Source: CAD feature listing. Evaluate the final solid. Frame: model axes, mm. A direction names the side the tool comes from. Coordinates: 2 decimals unless noted, no trailing zeros. Write each loop counter-clockwise with the first axis right and the second up, starting at its lowest first coordinate (ties: lowest second). Pieces come first, ordered by that corner, then holes. Notation, with made-up numbers: (48, -25.75) -> (87, -25.75) arc R9 ccw to (87, -12.75) -> close; hole circle Ø1 at (-33.5, 8). An arc over 180 degrees is marked (long way). One line per item, written item: value. Start each with the question number.
1. Line query: line 1 (Y direction, x = 10, z = 11); line 2 (X direction, y = 13.6, z = 0); line 3 (Z direction, x = 9, y = 7). Output: solid intervals per line, ascending.
2. First-contact query: P1, Ø2, axis at x = -3, z = 36.5, coming from the -Y side; P2, Ø7, axis at x = 0, z = 0, coming from the +Y side; P3, Ø5.5, axis at x = 3.5, z = 39, coming from the +Y side; P4, Ø4, axis at x = -9.5, y = 6.5, coming from the -Z side. Flat tips, straight axial feed; report the tip coordinate or a pass-through.
3. Section query A-A, the plane y = -0.5. Output: boundary loops of the cut face in (x, z), and give its area (3 significant figures).
4. Section query D-D, the plane z = -3. Output: boundary loops of the cut face in (x, y), and give its area (3 significant figures).
5. Section query B-B, the plane x = 0. Output: boundary loops of the cut face in (y, z), and give its area (3 significant figures).
6. Section query C-C, the plane z = -11. Output: boundary loops of the cut face in (x, y), and give its area (3 significant figures).
7. Access query for faces 4 (the flat face through (0, 12, 5)), 5 (the cylindrical face through (0, 0, 38)), 6 (the flat face through (-0.6, 4, 39.3)). Directions: +Z, -Z, +X, -X, +Y, -Y. A direction counts if a zero-diameter tool reaches every point of the face in a straight line with its end or side. Return the directions, or none.
8. Mould query, pull axis X, two halves, no side actions, for faces 1 (the flat face through (-0.6, -4, 39.3)), 2 (the cylindrical face through (0, 14, -15)), 3 (the cylindrical face through (-3.905, -13.972, -0.867)). Classes: released by +X, released by -X, zero draft, split by the parting line, or undercut.
from build123d import *

# Parameters (mm, degrees)
BOSS_EXTRUDE1_START = 12
SKETCH1_R           = 4
BOSS_EXTRUDE1_DEPTH = 4
BOSS_EXTRUDE2_START = -12
SKETCH1_2_R         = 4
BOSS_EXTRUDE2_DEPTH = 4
SKETCH2_W           = 30
SKETCH2_H           = 32
BOSS_EXTRUDE3_DEPTH = 8
BOSS_EXTRUDE4_START = -12
BOSS_EXTRUDE4_DEPTH = 8
FILLET1_R           = 1


with BuildPart() as part:
    # Sketch1 → Boss-Extrude1 (new body)
    with BuildSketch(Plane(origin=(0, 0, 0), x_dir=(1, 0, 0), z_dir=(0, 1, 0)).offset(BOSS_EXTRUDE1_START)):
        with BuildLine():
            Line((-15, 0), (-15, -25))
            Line((-15, -25), (15, -25))
            Line((15, -25), (15, 0))
            ThreePointArc((15, 0), (0, 15), (-15, 0))
        make_face()
        with Locations(Location((0, 0, 0), (0, 0, 270))):
            Circle(SKETCH1_R, mode=Mode.SUBTRACT)
    extrude(amount=BOSS_EXTRUDE1_DEPTH)



with BuildPart() as body_2:
    # Sketch1_2 → Boss-Extrude2 (new body)
    with BuildSketch(Plane(origin=(0, 0, 0), x_dir=(1, 0, 0), z_dir=(0, 1, 0)).offset(BOSS_EXTRUDE2_START)):
        with BuildLine():
            Line((-15, 0), (-15, -25))
            Line((-15, -25), (15, -25))
            Line((15, -25), (15, 0))
            ThreePointArc((15, 0), (0, 15), (-15, 0))
        make_face()
        with Locations(Location((0, 0, 0), (0, 0, 270))):
            Circle(SKETCH1_2_R, mode=Mode.SUBTRACT)
    extrude(amount=-BOSS_EXTRUDE2_DEPTH)


with BuildPart() as part_1:
    add(part.part)

    add(body_2.part)  # Boss-Extrude3 merges body 2
    # Sketch2 → Boss-Extrude3 (add)
    with BuildSketch(Plane.XY.offset(25)):
        Rectangle(SKETCH2_W, SKETCH2_H)
    extrude(amount=BOSS_EXTRUDE3_DEPTH)

    # Sketch3 → Boss-Extrude4 (add)
    with BuildSketch(Plane.XZ.offset(16).offset(BOSS_EXTRUDE4_START)):
        with BuildLine():
            ThreePointArc((9, 33), (0, 42), (-9, 33))
            Line((-9, 33), (-5, 33))
            ThreePointArc((-5, 33), (0, 38), (5, 33))
            Line((5, 33), (9, 33))
        make_face()
    extrude(amount=-BOSS_EXTRUDE4_DEPTH)

    # Fillet1
    fillet1_edges = [part_1.edges().sort_by_distance(p)[0] for p in [
        (7, -4, 33),
        (9, 0, 33),
        (0, -4, 38),
        (5, 0, 33),
        (-7, -4, 33),
        (-5, 0, 33),
        (0, 4, 42),
        (-9, 0, 33),
        (7, 4, 33),
        (0, 4, 38),
        (-7, 4, 33),
        (0, -4, 42),
    ]]
    fillet(fillet1_edges, radius=FILLET1_R)


solid = part_1.part
Computed values:
1. line 1: y = -16 to -12, 12 to 16
1. line 2: x = -15 to -4, 4 to 15
1. line 3: z = 25 to 33
2. P1: stops at y = -3.92
2. P2: passes through
2. P3: stops at y = 4
2. P4: stops at z = 25
3. outline: (-15, 25) -> (15, 25) -> (15, 33) -> (9.95, 33) arc R1 cw to (8.95, 33.9) arc R9 ccw to (-8.95, 33.9) arc R1 cw to (-9.95, 33) -> (-15, 33) -> close; hole (-4.84, 34.25) arc R1 ccw to (-3.87, 33) -> (3.87, 33) arc R1 ccw to (4.84, 34.25) arc R5 ccw to start
3. area: 329 mm²
4. outline: (-14.7, -16) -> (-2.65, -16) -> (-2.65, -12) -> (-14.7, -12) -> close; (-14.7, 12) -> (-2.65, 12) -> (-2.65, 16) -> (-14.7, 16) -> close; (2.65, -16) -> (14.7, -16) -> (14.7, -12) -> (2.65, -12) -> close; (2.65, 12) -> (14.7, 12) -> (14.7, 16) -> (2.65, 16) -> close
4. area: 193 mm²
5. outline: (-16, -15) -> (-12, -15) -> (-12, -4) -> (-16, -4) -> close; (-16, 4) -> (-12, 4) -> (-12, 25) -> (12, 25) -> (12, 4) -> (16, 4) -> (16, 33) -> (-16, 33) -> close; (-4, 39) arc R1 ccw to (-3, 38) -> (3, 38) arc R1 ccw to (4, 39) -> (4, 41) arc R1 ccw to (3, 42) -> (-3, 42) arc R1 ccw to (-4, 41) -> close; (12, -15) -> (16, -15) -> (16, -4) -> (12, -4) -> close
5. area: 543 mm²
6. outline: (-10.2, -16) -> (10.2, -16) -> (10.2, -12) -> (-10.2, -12) -> close; (-10.2, 12) -> (10.2, 12) -> (10.2, 16) -> (-10.2, 16) -> close
6. area: 163 mm²
7. face 4: -Z, +X, -X
7. face 5: +Y, -Y
7. face 6: +Z, +X, -X, +Y
8. face 1: zero draft
8. face 2: split by the parting line
8. face 3: undercut
